from build123d import *
from build123d.topology import SkipClean

# Parameters (mm, degrees)
RESSALTO_EXTRUS_O1_DEPTH      = 2.8
RESSALTO_EXTRUS_O1_DEPTH_BACK = 0.15
ESBO_O1_R                     = 3.6
ESBO_O1_R_2                   = 2.45
ESBO_O2_R                     = 2.5
ESBO_O2_R_2                   = 1
RESSALTO_EXTRUS_O2_DEPTH      = 0.5
ESBO_O3_R                     = 3.6
ESBO_O3_R_2                   = 2.45
RESSALTO_EXTRUS_O3_DEPTH      = 2.2
ESBO_O4_W                     = 22
ESBO_O4_H                     = 2.15
RESSALTO_EXTRUS_O4_DEPTH      = 3.6
CORTE_EXTRUS_O2_DEPTH         = 7.2
ESBO_O7_R                     = 2.5
CORTE_EXTRUS_O3_DEPTH         = 2.7
ESBO_O8_R                     = 1.5
ESBO_O8_R_2                   = 0.9
CORTE_EXTRUS_O4_DEPTH         = 6.9
RESSALTO_EXTRUS_O5_DEPTH      = 0.95
CORTE_EXTRUS_O5_DEPTH         = 12
CORTE_EXTRUS_O5_DEPTH_BACK    = 4.95


with BuildPart() as part:
    # Esbo_o1 → Ressalto-extrus_o1 (new, two sides: drawn at the far end of the back side and taken through both)
    with BuildSketch(Plane.XY.offset(-RESSALTO_EXTRUS_O1_DEPTH_BACK)):
        Circle(ESBO_O1_R)
        Circle(ESBO_O1_R_2, mode=Mode.SUBTRACT)
    extrude(amount=RESSALTO_EXTRUS_O1_DEPTH + RESSALTO_EXTRUS_O1_DEPTH_BACK)



with BuildPart() as body_2:
    # Esbo_o2 → Ressalto-extrus_o2 (new body)
    with BuildSketch(Plane(origin=(0, 0, -0.15), x_dir=(-1, 0, 0), z_dir=(0, 0, -1))):
        Circle(ESBO_O2_R)
        Circle(ESBO_O2_R_2, mode=Mode.SUBTRACT)
    extrude(amount=RESSALTO_EXTRUS_O2_DEPTH)


with BuildPart() as part_1:
    add(part.part)

    add(body_2.part)  # Ressalto-extrus_o3 merges body 2
    # Esbo_o3 → Ressalto-extrus_o3 (add)
    with BuildSketch(Plane(origin=(0, 0, -0.15), x_dir=(-1, 0, 0), z_dir=(0, 0, -1))):
        with Locations(Location((0, 0, 0), (0, 0, 180))):
            Circle(ESBO_O3_R)
        with Locations(Location((0, 0, 0), (0, 0, 180))):
            Circle(ESBO_O3_R_2, mode=Mode.SUBTRACT)
    extrude(amount=RESSALTO_EXTRUS_O3_DEPTH)

    # Esbo_o4 → Ressalto-extrus_o4 (add, symmetric)
    with BuildSketch(Plane(origin=(0, 0, 0), x_dir=(1, 0, 0), z_dir=(0, 1, 0))):
        with Locations((-7.325, 0.315)):
            Rectangle(ESBO_O4_W, ESBO_O4_H)
    extrude(amount=RESSALTO_EXTRUS_O4_DEPTH, both=True)

    # Esbo_o5 → Corte-extrus_o2 (cut)
    with SkipClean():  # the faces are left unmerged after this step: merging them gives an invalid solid
        with BuildSketch(Plane.XY.offset(0.76)):
            with BuildLine():
                ThreePointArc((0, -3.6), (-0.28434443, -3.588753021), (-0.566912184, -3.555082358))
                Line((-0.566912184, -3.555082358), (-16.183639111, -2.317736326))
                ThreePointArc((-16.183639111, -2.317736326), (-17.70771571, -1.577761723), (-18.325, -1.7e-08))
                Line((-18.325, -1.7e-08), (-18.325, -3.6))
                Line((-18.325, -3.6), (0, -3.6))
            make_face()
            with BuildLine():
                ThreePointArc((0, 3.6), (3.6, 0), (0, -3.6))
                Line((0, -3.6), (3.675, -3.6))
                Line((3.675, -3.6), (3.675, 3.6))
                Line((3.675, 3.6), (0, 3.6))
            make_face()
            with BuildLine():
                Line((-16.183639111, 2.317736326), (-0.566912184, 3.555082358))
                ThreePointArc((-0.566912184, 3.555082358), (-0.28434443, 3.588753021), (0, 3.6))
                Line((0, 3.6), (-18.325, 3.6))
                Line((-18.325, 3.6), (-18.325, -1.7e-08))
                ThreePointArc((-18.325, -1.7e-08), (-17.707715722, 1.57776171), (-16.183639111, 2.317736326))
            make_face()
        extrude(amount=-CORTE_EXTRUS_O2_DEPTH, mode=Mode.SUBTRACT)

    # Esbo_o7 → Corte-extrus_o3 (cut)
    with SkipClean():  # the faces are left unmerged after this step: merging them gives an invalid solid
        with BuildSketch(Plane.XY.offset(2.8)):
            Circle(ESBO_O7_R)
        extrude(amount=-CORTE_EXTRUS_O3_DEPTH, mode=Mode.SUBTRACT)

    # Esbo_o8 → Corte-extrus_o4 (cut, symmetric)
    with BuildSketch(Plane.XY.offset(0.1)):
        Circle(ESBO_O8_R)
        with Locations((-6, 0)):
            Circle(ESBO_O8_R_2)
        with Locations((-8.5, 0)):
            Circle(ESBO_O8_R_2)
        with Locations((-11, 0)):
            Circle(ESBO_O8_R_2)
        with Locations((-13.5, 0)):
            Circle(ESBO_O8_R_2)
        with Locations((-16, 0)):
            Circle(ESBO_O8_R_2)
    extrude(amount=CORTE_EXTRUS_O4_DEPTH, both=True, mode=Mode.SUBTRACT)

    # Esbo_o10 → Ressalto-extrus_o5 (add)
    with BuildSketch(Plane(origin=(0, 0, -1.39), x_dir=(-1, 0, 0), z_dir=(0, 0, -1))):
        with BuildLine():
            Line((0.566912184, -3.555082358), (5.1, -3.195916302))
            Line((5.1, -3.195916302), (5.1, -2.395916302))
            Line((5.1, -2.395916302), (2.686928558, -2.395916302))
            ThreePointArc((2.686928558, -2.395916302), (1.727074515, -3.158672763), (0.566912184, -3.555082358))
        make_face()
        with BuildLine():
            ThreePointArc((3.577708764, 0.4), (3.6, 0), (3.577708764, -0.4))
            Line((3.577708764, -0.4), (5.193774225, -0.4))
            ThreePointArc((5.193774225, -0.4), (5.1, 0), (5.193774225, 0.4))
            Line((5.193774225, 0.4), (3.577708764, 0.4))
        make_face()
        with BuildLine():
            ThreePointArc((0.566912184, 3.555082358), (1.727074515, 3.158672763), (2.686928558, 2.395916302))
            Line((2.686928558, 2.395916302), (5.1, 2.395916302))
            Line((5.1, 2.395916302), (5.1, 3.195916302))
            Line((5.1, 3.195916302), (0.566912184, 3.555082358))
        make_face()
    extrude(amount=RESSALTO_EXTRUS_O5_DEPTH)

    # Esbo_o11 → Corte-extrus_o5 (cut, two sides: drawn at the far end of the back side and taken through both)
    with BuildSketch(Plane(origin=(0, 0, 0), x_dir=(1, 0, 0), z_dir=(0, 1, 0)).offset(-CORTE_EXTRUS_O5_DEPTH_BACK)):
        Polygon((-5.1, 1.39), (-2.045555334, 3.15348445), (-5.859008957, 3.15348445), (-5.859008957, 1.39), align=None)
    extrude(amount=CORTE_EXTRUS_O5_DEPTH + CORTE_EXTRUS_O5_DEPTH_BACK, mode=Mode.SUBTRACT)

    # Espelhar20: part across plane


with BuildPart() as part_2:
    with SkipClean():  # the faces are left unmerged after this step: merging them gives an invalid solid
        add(part_1.part)
        add(part_1.part.mirror(Plane.ZY))
    add(part_2.part.scale(1), mode=Mode.REPLACE)  # the faces are merged on a copy


solid = part_2.part
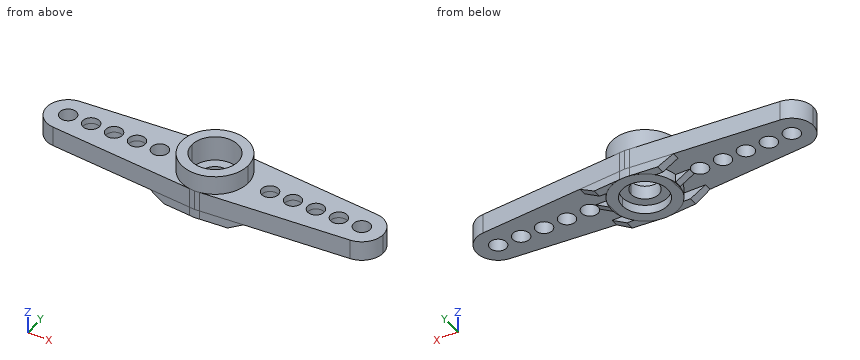
CAD build for the part. Positions are in the model's coordinates, mm. Give positions to 0.01 mm unless a question says otherwise; leave off trailing zeros. Loops run counter-clockwise (first coordinate to the right, second up) from the corner with the lowest first, then second, coordinate; pieces in that order, holes last. Notation, with made-up numbers: M 82,12 L 133,12 A35 ccw 133,44 Z; hole C 53.5,69 d10. An arc over 180 degrees is marked long. One line per question, with ' | ' between items. Start each with the question number.
1. Flat gauge pins, fed straight in: pin 1 (1 mm diameter, centred on x = -4, z = -2, fed in from +Y); pin 2 (3 mm diameter, centred on x = 11, y = 0, fed in from -Z); pin 3 (0.8 mm diameter, centred on x = -3.5, z = -1.5, fed in from -Y). Where does each tip first touch, or does it go through?
2. Saw through at C-C on x = 8.5. Give the cut face in (y, z).
3. Saw through at A-A on x = -6. Give the cut face in (y, z).
4. Saw through at B-B on z = 1.55. Give the cut face in (x, y), plus the area to 3 significant figures.
5. Probe L1, parallel to Z at x = 15, y = -2; L2, parallel to Y at x = -6, z = -0.35; L3, parallel to Y at x = 14.5, z = 0.05. List the from-to ranges inside material, lowest first. Write a range as from..to.
Result sheet:
1) pin 1: stops at y = 3.32 | pin 2: stops at z = -1.39 | pin 3: stops at y = -3.35
2) outline: M -2.93,-1.39 L -0.9,-1.39 L -0.9,0.76 L -2.93,0.76 Z; M 0.9,-1.39 L 2.93,-1.39 L 2.93,0.76 L 0.9,0.76 Z
3) outline: M -3.12,-1.39 L -0.9,-1.39 L -0.9,0.76 L -3.12,0.76 Z; M 0.9,-1.39 L 3.12,-1.39 L 3.12,0.76 L 0.9,0.76 Z
4) outline: C 0,0 d7.2; hole C 0,0 d5 | area: 21.1 mm^2
5) L1: z = -1.39..0.76 | L2: y = -3.12..-0.9, 0.9..3.12 | L3: y = -2.45..2.45
